from build123d import *

# Parameters (mm, degrees)
F1_R     = 4.25
F3_DEPTH = 25
F4_SIZE  = 3.99999


# Not quite as in the source:
# - a fillet or chamfer is up to 0.001 mm smaller than in the source, because OpenCascade refuses the exact size


with BuildPart() as f2:
    # F0 (on Front) → F2 (revolve)
    with BuildSketch(Plane.XZ):
        Polygon((0, 4), (0, 0), (34, 0), (34, 35), (30.5, 35), (30.5, 4), align=None)
    revolve(axis=Axis((0, 0, 2), (0, 0, -1)))

    # F1 (on Top) → F3 (cut)
    with BuildSketch(Plane.XY):
        with Locations((-10.5, -18.1865334795)):
            Circle(F1_R)
        with Locations((-10.5, 18.1865334795)):
            Circle(F1_R)
        with Locations((21, 0)):
            Circle(F1_R)
    extrude(amount=F3_DEPTH, mode=Mode.SUBTRACT)

    # F4 (size 4 in the source; OpenCascade refuses exactly that, so slightly less here)
    f4_edges = [f2.edges().sort_by_distance(p)[0] for p in [
        (16.75, 0, 4),
        (-14.75, 18.186533, 4),
        (-14.75, -18.186533, 4),
    ]]
    chamfer(f4_edges, length=F4_SIZE)


solid = f2.part
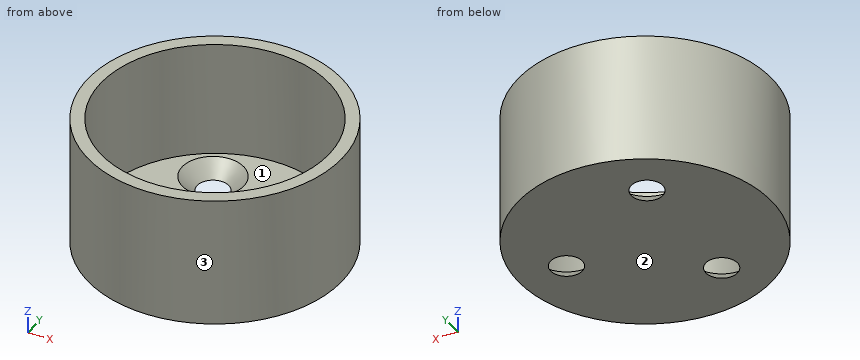
Input: part model. Units: mm. Frame: model coordinates. Face numbers are marked on the shaded views. Round coordinates to 2 decimals unless told otherwise and drop trailing zeros. Write each loop counter-clockwise with the first axis right and the second up, starting at its lowest first coordinate (ties: lowest second). Pieces come first, ordered by that corner, then holes.
1) Cut plane D-D (x = -10.5). Count the separate pieces of the cut face and the enclosed holes in it, then the cut area to 3 significant figures.
2) Contact query for flat-ended pins moving along their axis: P1, Ø8, axis at y = 9.5, z = 7, coming from the -X side; P2, Ø3, axis at x = -6.5, z = 8.5, coming from the -Y side; P3, Ø4, axis at x = -21, y = -7.5, coming from the +Z side. Output: stop coordinate, or through.
3) Cut plane C-C (z = 27). Return the cut outline in (x, y).
4) Draft query along Y for the marked faces 1, 2 and 3. Return one class per face: pulls with the +Y half, pulls with the -Y half, needs draft (parallel to the pull), parting line crosses it, or undercut.
5) Ray query, L1, parallel to Y at x = -10.5, z = 0.05; L2, parallel to X at y = 0, z = 11; L3, parallel to Y at x = -1, z = 14. Return the intervals inside material, ascending.
6) Cut plane B-B (x = 0). Return the cut outline in (y, z).
Geometry says:
1. separate pieces: 3
1. enclosed holes: 0
1. area: 388 mm2
2. P1: stops at x = -33.55
2. P2: stops at y = -33.63
2. P3: stops at z = 4
3. outline: circle Ø68 at (0, 0); hole circle Ø61 at (0, 0)
4. face 1: undercut
4. face 2: needs draft
4. face 3: parting line crosses it
5. L1: y = -32.34 to -22.49, -13.89 to 13.89, 22.49 to 32.34
5. L2: x = -34 to -30.5, 30.5 to 34
5. L3: y = -33.99 to -30.48, 30.48 to 33.99
6. outline: (-34, 0) - (34, 0) - (34, 35) - (30.5, 35) - (30.5, 4) - (-30.5, 4) - (-30.5, 35) - (-34, 35) - close
